from build123d import *

# Parameters (mm, degrees)
EXTRUDE_1_DEPTH             = 60
SKETCH_2_R                  = 2
EXTRUDE_2_DEPTH             = 15
SKETCH_3_R                  = 2
SKETCH_3_R_2                = 1.6
CUT_EXTRUDE_3_DEPTH         = 0.5
CHAMFER_1_SIZE              = 0.4
HOLE_WIZARD_M31_D           = 2.2
HOLE_WIZARD_M31_DEPTH       = 8
HOLE_WIZARD_M31_CSINK_D     = 3
HOLE_WIZARD_M31_CSINK_ANGLE = 90
HOLE_WIZARD_M31_TIP         = 0.660946681


with BuildPart() as part:
    # Эскиз1 → Вытянуть1 (new body)
    with BuildSketch(Plane.XY):
        Polygon((0, 4.041451884), (-3.5, 2.020725942), (-3.5, -2.020725942), (0, -4.041451884), (3.5, -2.020725942), (3.5, 2.020725942), align=None)
    extrude(amount=EXTRUDE_1_DEPTH)

    # Эскиз2 → Вытянуть2 (add)
    with BuildSketch(Plane.XY.offset(60)):
        Circle(SKETCH_2_R)
    extrude(amount=EXTRUDE_2_DEPTH)

    # Эскиз3 → Вырез-Вытянуть3 (cut)
    with BuildSketch(Plane.XY.offset(60)):
        Circle(SKETCH_3_R)
        Circle(SKETCH_3_R_2, mode=Mode.SUBTRACT)
    extrude(amount=CUT_EXTRUDE_3_DEPTH, mode=Mode.SUBTRACT)

    # Фаска1
    chamfer_1_edges = [part.edges().sort_by_distance(p)[0] for p in [
        (-2, 0, 75),
        (-2, 0, 60.5),
    ]]
    chamfer(chamfer_1_edges, length=CHAMFER_1_SIZE - 0.0001)  # a hair under: the kernel refuses the full size

    # Отверстие с зазором M31
    with Locations(Plane(origin=(0, 0, 0), x_dir=(-1, 0, 0), z_dir=(0, 0, -1))):
        with Locations((0, 0)):
            CounterSinkHole(HOLE_WIZARD_M31_D / 2, HOLE_WIZARD_M31_CSINK_D / 2, depth=HOLE_WIZARD_M31_DEPTH, counter_sink_angle=HOLE_WIZARD_M31_CSINK_ANGLE)
            with Locations((0, 0, -(HOLE_WIZARD_M31_DEPTH + HOLE_WIZARD_M31_TIP / 2))):  # 118° drill point
                Cone(0, HOLE_WIZARD_M31_D / 2, HOLE_WIZARD_M31_TIP, mode=Mode.SUBTRACT)


solid = part.part
Geometry: final body of the model. Coordinates: model frame, mm. A direction names the side the tool comes from. Coordinates: 2 decimals unless noted, no trailing zeros. Order: outer loops, then holes, each group sorted by start corner. A loop starts at its lowest first (then second) coordinate and runs counter-clockwise, first axis right, second up.
(1) Section query D-D (x = 2.75). Return the cut outline in (y, z), plus the area to 3 significant figures.
(2) Access query for faces 5 (the face through (-1.8, -3, 29.6)), 6 (the face through (0, -2, 68)), 7 (the face through (-2, 0, 60)). Directions: +Z, -Z, +X, -X, +Y, -Y. A direction counts if a zero-diameter tool reaches every point of the face in a straight line with its end or side. Return the directions, or none.
(3) Material intervals for probe 1 along Y at (x, z) = (0, 2.5); probe 2 along X at (y, z) = (0, 2.5); probe 3 along Z at (x, y) = (1, 2.5), sorted ascending.
(4) Section query B-B (z = 42). Return the cut outline in (x, y).
(5) First-contact query: pin 1 (1 mm diameter, centred on x = -1, z = 7.5, fed in from +Y); pin 2 (1 mm diameter, centred on y = -3, z = 16.5, fed in from +X). Flat tips, straight axial feed; report the tip coordinate or a pass-through.
(6) Draft query along X for faces 1 (the face through (0.041, -0.186, 8.546)), 2 (the face through (1.05, 0.33, 4.25)), 3 (the face through (1.8, 3, 29.6)), 4 (the face through (-1.27, -0.97, 60.25)). Return one class per face: pulls with the +X half, pulls with the -X half, needs draft (parallel to the pull), parting line crosses it, or undercut.
(7) Section query A-A (z = 5). Return the cut outline in (x, y).
(8) Section query C-C (y = -2.75). Return the cut outline in (x, z), plus the area to 3 significant figures.
Solution:
1. outline: (-2.45, 0) - (2.45, 0) - (2.45, 60) - (-2.45, 60) - close
1. area: 294 mm2
2. face 5: +Z, -Z, -X, -Y
2. face 6: +Z
2. face 7: none
3. probe 1: y = -4.04 to -1.1, 1.1 to 4.04
3. probe 2: x = -3.5 to -1.1, 1.1 to 3.5
3. probe 3: z = 0 to 60
4. outline: (-3.5, -2.02) - (0, -4.04) - (3.5, -2.02) - (3.5, 2.02) - (0, 4.04) - (-3.5, 2.02) - close
5. pin 1: stops at y = 3.75
5. pin 2: stops at x = 2.67
6. face 1: undercut
6. face 2: undercut
6. face 3: pulls with the +X half
6. face 4: parting line crosses it
7. outline: (-3.5, -2.02) - (0, -4.04) - (3.5, -2.02) - (3.5, 2.02) - (0, 4.04) - (-3.5, 2.02) - close; hole circle Ø2.2 at (0, 0)
8. outline: (-2.24, 0) - (2.24, 0) - (2.24, 60) - (-2.24, 60) - close
8. area: 268 mm2
